from build123d import *

# Parameters (mm, degrees)
F1_DEPTH = 5


# Not quite as in the source:
# - ends of sketch curves that miss each other by under 0.0002 mm in the source are joined


with BuildPart() as f1:
    # F0 (on Front) → F1 (new body)
    with BuildSketch(Plane.XZ):
        with BuildLine():
            Line((-8.2946076301, 0), (-10.7946076301, 0))
            ThreePointArc((-10.7946076301, 0), (4.2053923699, -15), (19.2053923699, 0))
            Line((19.2053923699, 0), (16.705392798, 0.0014630326))
            ThreePointArc((16.705392798, 0.0014630326), (4.2061241002, -12.4992684623), (-8.2946076301, 0))
        make_face()
        with BuildLine():
            ThreePointArc((-40.7946076301, 0), (-25.7946076301, 15), (-10.7946076301, 0))
            Line((-10.7946076301, 0), (-8.2946076301, 0))
            ThreePointArc((-8.2946076301, 0), (-25.7946076301, 17.5), (-43.2946076301, 0))
            Line((-43.2946076301, 0), (-40.7946076301, 0))
        make_face()
        with BuildLine():
            ThreePointArc((-70.7936146824, 0), (-55.7941111563, -15.1220408499), (-40.7946076301, 0))
            Line((-40.7946076301, 0), (-43.2946076301, 0))
            ThreePointArc((-43.2946076301, 0), (-55.7941111563, -12.6114073597), (-68.2936146824, 0))
            Line((-68.2936146824, 0), (-70.7936146824, 0))
        make_face()
        with BuildLine():
            Line((16.705392798, 0.0014630326), (19.2053923699, 0))
            ThreePointArc((19.2053923699, 0), (34.2052637046, 14.9378715725), (49.2051350393, 0))
            Line((49.2051350393, 0), (51.7051350393, 0))
            ThreePointArc((51.7051350393, 0), (34.205992633, 17.4335732975), (16.705392798, 0.0014630326))
        make_face()
        with BuildLine():
            Line((51.7051350393, 0), (49.2051350393, 0))
            ThreePointArc((49.2051350393, 0), (50.4551350393, -0.0521740711), (51.7051350393, 0))
        make_face()
        with BuildLine():
            ThreePointArc((51.7051350393, 0), (50.4551350393, -0.0521740711), (49.2051350393, 0))
            ThreePointArc((49.2051350393, 0), (64.205134968, -14.9985369674), (79.2051348966, 0))
            Line((79.2051348966, 0), (76.7051348966, 0))
            ThreePointArc((76.705134968, 0), (64.205134968, -12.5), (51.705134968, 0))
        make_face()
    extrude(amount=F1_DEPTH)


solid = f1.part
Geometry check sheet. Reference: the model listing, model coordinates, mm. A direction names the side the tool comes from. Give positions to 0.01 mm unless a question says otherwise; leave off trailing zeros. Order: outer loops, then holes, each group sorted by start corner. A loop starts at its lowest first (then second) coordinate and runs counter-clockwise, first axis right, second up. Notation, with made-up numbers: (-13.75, -4) - (4.25, -4) arc R19 cw to (4.25, 26) - close; hole circle Ø3 at (6.25, 73.25). An arc over 180 degrees is marked (long way). Answer as a JSON object with one key per item and string values.
(1) Cross-section at C-C (y = -3.1). Record the cut outline in (x, z).
Report:
{"outline": "(-70.79, 0) arc R15 ccw (long way) to (-40.79, 0) arc R15 cw to (-10.79, 0) arc R15 ccw to (19.21, 0) arc R15 cw to (49.21, 0) arc R15 ccw to (79.21, 0) - (76.71, 0) arc R12.5 cw to (51.71, 0) arc R17.5 ccw to (16.71, 0) arc R12.5 cw to (-8.29, 0) arc R17.5 ccw to (-43.29, 0) arc R12.5 cw (long way) to (-68.29, 0) - close"}
(2) Draft check along X on faces 3 (the cylindrical face through (-55.52, -2.46, -12.61)), 4 (the flat face through (78, -2, 0)). Enter one of: released by +X, released by -X, zero draft, split by the parting line, or undercut.
Report:
{"face 3": "undercut", "face 4": "zero draft"}
(3) Cross-section at B-B (z = -6). Record the cut outline in (x, y), then the cut area to 3 significant figures.
Report:
{"outline": "(-69.59, -5) - (-66.82, -5) - (-66.82, 0) - (-69.59, 0) - close; (-44.77, -5) - (-41.99, -5) - (-41.99, 0) - (-44.77, 0) - close; (-9.54, -5) - (-6.76, -5) - (-6.76, 0) - (-9.54, 0) - close; (15.17, -5) - (17.95, -5) - (17.95, 0) - (15.17, 0) - close; (50.46, -5) - (53.24, -5) - (53.24, 0) - (50.46, 0) - close; (75.17, -5) - (77.95, -5) - (77.95, 0) - (75.17, 0) - close", "area": "83.4 mm^2"}
(4) Material ranges on line 1 (X direction, y = -3.5, z = -7.5); line 2 (X direction, y = -2.35, z = -9); line 3 (X direction, y = -2.9, z = 11), recorded low to high.
Report:
{"line 1": "-68.85 to -65.88, -45.71 to -42.73, -8.78 to -5.79, 14.2 to 17.2, 51.22 to 54.21, 74.21 to 77.19", "line 2": "-67.88 to -64.58, -47.01 to -43.7, -7.79 to -4.47, 12.88 to 16.21, 52.21 to 55.53, 72.88 to 76.2", "line 3": "-39.41 to -35.99, -15.6 to -12.18, 20.65 to 24.07, 44.34 to 47.76"}
(5) Cross-section at A-A (z = 13.5). Record the cut outline in (x, y).
Report:
{"outline": "(-36.93, -5) - (-32.33, -5) - (-32.33, 0) - (-36.93, 0) - close; (-19.26, -5) - (-14.66, -5) - (-14.66, 0) - (-19.26, 0) - close; (23.15, -5) - (27.8, -5) - (27.8, 0) - (23.15, 0) - close; (40.61, -5) - (45.26, -5) - (45.26, 0) - (40.61, 0) - close"}
(6) Depth check by flat-ended pin: pin 1 Ø1 at (y, z) = (-4, -8.5) entering from -X; pin 2 Ø1.2 at (x, y) = (-69.5, -2) entering from +Z; pin 3 Ø3 at (y, z) = (-3.5, -5.5) entering from -X. Enter the tip coordinate at first touch or a pass-through.
Report:
{"pin 1": "x = -68.56", "pin 2": "z = 0", "pin 3": "x = -70.28"}
(7) Tool access check on faces 1 (the flat face through (-7, 0, -6)), 2 (the flat face through (-70, -2, 0)). Record the directions out of +Z, -Z, +X, -X, +Y, -Y that give a thin tool (end or side, any length) a straight path to the whole face; none if there is none.
Report:
{"face 1": "+Z, -Z, +X, -X, +Y", "face 2": "+Z, -X, +Y, -Y"}
(8) Cross-section at D-D (z = 6.5). Record the cut outline in (x, y), then the cut area to 3 significant figures.
Report:
{"outline": "(-42.04, -5) - (-39.31, -5) - (-39.31, 0) - (-42.04, 0) - close; (-12.28, -5) - (-9.55, -5) - (-9.55, 0) - (-12.28, 0) - close; (17.98, -5) - (20.72, -5) - (20.72, 0) - (17.98, 0) - close; (47.69, -5) - (50.43, -5) - (50.43, 0) - (47.69, 0) - close", "area": "54.6 mm^2"}
